Geometry: final body of the model. Coordinates: model frame, mm. A direction names the side the tool comes from. Give positions to 0.01 mm unless a question says otherwise; leave off trailing zeros. Write each loop counter-clockwise with the first axis right and the second up, starting at its lowest first coordinate (ties: lowest second). Pieces come first, ordered by that corner, then holes.
Q1. Section B-B (z = 0). Return the cut outline in (x, y).
Q2. Reachability of faces 1 (the flat face through (42, 0, 8)), 2 (the flat face through (-40, 6, -34)), 3 (the flat face through (-1, 0, 37)), 4 (the flat face through (-49, 20.5, 2)), 5 (the flat face through (-1, 0, -37)) from +Z, -Z, +X, -X, +Y, -Y: full face, straight path, thin tool, end or side. Return the list, or none.
Q3. Section D-D (x = 0). Return the cut outline in (y, z), plus the area to 3 significant figures.
Q4. Section A-A (x = -61). Return the cut outline in (y, z).
Q5. Pin query (flat end, axial travel): pin 1 Ø13.5 at (x, y) = (5, 14) entering from +Z; pin 2 Ø3 at (x, y) = (-33, 9) entering from +Z; pin 3 Ø3 at (x, z) = (-10, 30.5) entering from +Y. Return the tip coordinate at first contact, or that it passes through.
Q6. Line query: line 1 (Z direction, x = 0, y = 20.9); line 2 (X direction, y = 20, z = 13); line 3 (Y direction, x = 38.5, z = -2.5). Output: solid intervals per line, ascending.
Q7. Mould query, pull axis Z, two halves, no side actions, for faces 6 (the flat face through (-70.176, 20, 0)), 7 (the cylindrical face through (-25.756, 11.154, 34.425)), 8 (the flat face through (41, 22, 0)). Classes: +Z half, -Z half, draft (parallel to the pull), parting line (faces both ways), or undercut.
Q8. Section C-C (y = 7). Return the cut outline in (x, z), plus the area to 3 significant figures.
from build123d import *

# Parameters (mm, degrees)
BOSS_EXTRUDE1_DEPTH = 22
FILLET1_R           = 10
CUT_EXTRUDE1_DEPTH  = 3.5
FILLET2_R           = 10
SKETCH4_W           = 17.500655667
SKETCH4_H           = 34.508335117
BOSS_EXTRUDE2_DEPTH = 2
SKETCH5_W           = 113.192264834
SKETCH5_H           = 68
BOSS_EXTRUDE3_DEPTH = 5


with BuildPart() as part:
    # Sketch1 → Boss-Extrude1 (new body)
    with BuildSketch(Plane(origin=(0, 0, 0), x_dir=(1, 0, 0), z_dir=(0, 1, 0))):
        with BuildLine():
            Line((-70.5, 34), (-25.5, 34))
            ThreePointArc((-25.5, 34), (42.5, 0), (-25.5, -34))
            Line((-25.5, -34), (-70.5, -34))
            Line((-70.5, -34), (-70.5, 34))
        make_face()
    extrude(amount=BOSS_EXTRUDE1_DEPTH)

    # Fillet1
    fillet1_edges = [part.edges().sort_by_distance(p)[0] for p in [
        (-25.5, 11, -34),
        (-25.5, 11, 34),
    ]]
    fillet(fillet1_edges, radius=FILLET1_R)

    # Sketch3 → Cut-Extrude1 (cut)
    with BuildSketch(Plane(origin=(0, 22, 0), x_dir=(1, 0, 0), z_dir=(0, 1, 0))):
        with BuildLine():
            Line((-22.471845342, 33.091028496), (-70.175642943, 33.091028496))
            Line((-70.175642943, 33.091028496), (-70.175642943, -33.21427255))
            Line((-70.175642943, -33.21427255), (-22.289282155, -33.21427255))
            ThreePointArc((-22.289282155, -33.21427255), (39.99984838, 0.110134479), (-22.471845342, 33.091028496))
        make_face()
    extrude(amount=-CUT_EXTRUDE1_DEPTH, mode=Mode.SUBTRACT)

    # Fillet2
    fillet2_edges = [part.edges().sort_by_distance(p)[0] for p in [
        (-22.471845342, 20.25, -33.091028496),
        (-22.289282155, 20.25, 33.21427255),
    ]]
    fillet(fillet2_edges, radius=FILLET2_R)

    # Sketch4 → Boss-Extrude2 (add)
    with BuildSketch(Plane(origin=(0, 18.5, 0), x_dir=(1, 0, 0), z_dir=(0, 1, 0))):
        with Locations((-48.878067279, -2.156770944)):
            Rectangle(SKETCH4_W, SKETCH4_H)
    extrude(amount=BOSS_EXTRUDE2_DEPTH)

    # Sketch5 → Boss-Extrude3 (add)
    with BuildSketch(Plane.XZ):
        with Locations((-13.903867583, 0)):
            Rectangle(SKETCH5_W, SKETCH5_H)
    extrude(amount=BOSS_EXTRUDE3_DEPTH)


solid = part.part
Computed:
1. outline: (-70.5, -5) - (42.69, -5) - (42.69, 0) - (42.5, 0) - (42.5, 22) - (40, 22) - (40, 18.5) - (-40.13, 18.5) - (-40.13, 20.5) - (-57.63, 20.5) - (-57.63, 18.5) - (-70.18, 18.5) - (-70.18, 22) - (-70.5, 22) - close
2. face 1: +X, +Y
2. face 2: -Z, -X, -Y
2. face 3: +Z, +X, -X, -Y
2. face 4: +Y
2. face 5: -Z, +X, -X, -Y
3. outline: (-5, -34) - (0, -34) - (0, -42.5) - (22, -42.5) - (22, -40) - (18.5, -40) - (18.5, 40) - (22, 40) - (22, 42.5) - (0, 42.5) - (0, 34) - (-5, 34) - close
3. area: 1,930 mm2
4. outline: (-5, -34) - (22, -34) - (22, -33.09) - (18.5, -33.09) - (18.5, 33.21) - (22, 33.21) - (22, 34) - (-5, 34) - close
5. pin 1: stops at z = 42.5
5. pin 2: stops at z = 34
5. pin 3: stops at y = 18.5
6. line 1: z = -42.5 to -40, 40 to 42.5
6. line 2: x = -70.5 to -70.18, -57.63 to -40.13, 37.83 to 40.46
6. line 3: y = -5 to 18.5
7. face 6: undercut
7. face 7: +Z half
7. face 8: draft
8. outline: (-70.5, -34) - (-28.64, -34) arc R10 cw to (-23.18, -35.62) arc R42.5 ccw (long way) to (-23.18, 35.62) arc R10 cw to (-28.64, 34) - (-70.5, 34) - close
8. area: 7,930 mm2
